The listing builds one solid part. Answer for the finished solid, in the listing's coordinates (mm). A direction names the side the tool comes from. Give positions to 0.01 mm unless a question says otherwise; leave off trailing zeros. Order: outer loops, then holes, each group sorted by start corner. A loop starts at its lowest first (then second) coordinate and runs counter-clockwise, first axis right, second up. Notation, with made-up numbers: (-39.5, 17) - (0.5, 17) arc R31 ccw to (0.5, 56) - close; hole circle Ø11 at (33.25, 18). An arc over 180 degrees is marked (long way). Answer in a Markdown table with one row per item.
from build123d import *

# Parameters (mm, degrees)
F0_W     = 80
F0_H     = 67
F0_R     = 2.5
F0_R_2   = 5
F0_R_3   = 4
F0_R_4   = 3.25
F1_DEPTH = 11.5
F2_SIZE2 = 3
F2_SIZE  = 3
F3_R     = 5
F3_R_2   = 3.25
F4_DEPTH = 5.5


with BuildPart() as f1:
    # F0 (on Top) → F1 (new body)
    with BuildSketch(Plane.XY):
        with Locations((40, 33.5)):
            Rectangle(F0_W, F0_H)
        with Locations((10, 10)):
            Circle(F0_R, mode=Mode.SUBTRACT)
        with Locations((20, 10)):
            Circle(F0_R, mode=Mode.SUBTRACT)
        with Locations((30, 10)):
            Circle(F0_R, mode=Mode.SUBTRACT)
        with Locations((12, 25)):
            Circle(F0_R_2, mode=Mode.SUBTRACT)
        with Locations((26, 25)):
            Circle(F0_R_3, mode=Mode.SUBTRACT)
        with Locations((40, 10)):
            Circle(F0_R, mode=Mode.SUBTRACT)
        with Locations((50, 10)):
            Circle(F0_R, mode=Mode.SUBTRACT)
        with Locations((60, 10)):
            Circle(F0_R, mode=Mode.SUBTRACT)
        with Locations((70, 10)):
            Circle(F0_R, mode=Mode.SUBTRACT)
        with Locations((40, 25)):
            Circle(F0_R_2, mode=Mode.SUBTRACT)
        with BuildLine():
            Line((54, 29), (70, 29))
            ThreePointArc((70, 29), (74, 25), (70, 21))
            Line((70, 21), (54, 21))
            ThreePointArc((54, 21), (50, 25), (54, 29))
        make_face(mode=Mode.SUBTRACT)
        with Locations((10, 42)):
            Circle(F0_R_3, mode=Mode.SUBTRACT)
        with Locations((21, 42)):
            Circle(F0_R_3, mode=Mode.SUBTRACT)
        with Locations((35, 42)):
            Circle(F0_R_4, mode=Mode.SUBTRACT)
        with Locations((10, 57)):
            Circle(F0_R, mode=Mode.SUBTRACT)
        with Locations((20, 57)):
            Circle(F0_R, mode=Mode.SUBTRACT)
        with Locations((30, 57)):
            Circle(F0_R, mode=Mode.SUBTRACT)
        with Locations((52, 42)):
            Circle(F0_R_3, mode=Mode.SUBTRACT)
        with Locations((69, 42)):
            Circle(F0_R_2, mode=Mode.SUBTRACT)
        with Locations((40, 57)):
            Circle(F0_R, mode=Mode.SUBTRACT)
        with Locations((50, 57)):
            Circle(F0_R, mode=Mode.SUBTRACT)
        with Locations((60, 57)):
            Circle(F0_R, mode=Mode.SUBTRACT)
        with Locations((70, 57)):
            Circle(F0_R, mode=Mode.SUBTRACT)
    extrude(amount=F1_DEPTH)

    # F2
    f2_edges = [f1.edges().sort_by_distance(p)[0] for p in [
        (31.75, 42, 11.5),
    ]]
    chamfer(f2_edges, length=F2_SIZE, length2=F2_SIZE2)

    # F3 (on face) → F4 (join)
    with BuildSketch(Plane(origin=(0, 0, 0), x_dir=(1, 0, 0), z_dir=(0, 0, -1))):
        with Locations((40, -25)):
            Circle(F3_R)
        with Locations((40, -25)):
            Circle(F3_R_2, mode=Mode.SUBTRACT)
    extrude(amount=-F4_DEPTH)


solid = f1.part
Item 1: Find section D-D on y = 42. Write down the section's boundary in (x, z).
Answer block:
| item | result |
|---|---|
| outline | (0, 0) - (6, 0) - (6, 11.5) - (0, 11.5) - close; (14, 0) - (17, 0) - (17, 11.5) - (14, 11.5) - close; (25, 0) - (31.75, 0) - (31.75, 8.5) - (28.75, 11.5) - (25, 11.5) - close; (38.25, 0) - (48, 0) - (48, 11.5) - (41.25, 11.5) - (38.25, 8.5) - close; (56, 0) - (64, 0) - (64, 11.5) - (56, 11.5) - close; (74, 0) - (80, 0) - (80, 11.5) - (74, 11.5) - close |
Item 2: This flat-tipped pin is pushed along its axis until it touches: P1, Ø10, axis at x = 13, y = 40, coming from the -Z side. Where does it stop, or does it pass through?
Answer block:
| item | result |
|---|---|
| P1 | z = 0 |
Item 3: Consider line 1 (Y direction, x = 40, z = 3.25); line 2 (Y direction, x = 66, z = 4); line 3 (Y direction, x = 26, z = 5.25). Determine where each line is inside the solid, lowest interval first.
Answer block:
| item | result |
|---|---|
| line 1 | 0 to 7.5, 12.5 to 21.75, 28.25 to 54.5, 59.5 to 67 |
| line 2 | 0 to 21, 29 to 38, 46 to 67 |
| line 3 | 0 to 21, 29 to 67 |
Item 4: Find section B-B on x = 15.5. Write down the section's boundary in (y, z).
Answer block:
| item | result |
|---|---|
| outline | (0, 0) - (21.43, 0) - (21.43, 11.5) - (0, 11.5) - close; (28.57, 0) - (67, 0) - (67, 11.5) - (28.57, 11.5) - close |
Item 5: Which of the six approach directions +Z, -Z, +X, -X, +Y, -Y give full straight-line access (tool end or side, diameter ignored) to faces 4 (the face through (50, 25, 6)), 5 (the face through (39, 34, 11.5))?
Answer block:
| item | result |
|---|---|
| face 4 | +Z, -Z |
| face 5 | +Z, +X, -X, +Y, -Y |
Item 6: Determine the mould class of faces 1 (the face through (39, 67, 6)), 2 (the face through (17.5, 57.1, 5.7)), 3 (the face through (80, 33, 6)) for opening direction X: pulls with the +X half, pulls with the -X half, needs draft (parallel to the pull), parting line crosses it, or undercut.
Answer block:
| item | result |
|---|---|
| face 1 | needs draft |
| face 2 | undercut |
| face 3 | pulls with the +X half |
Item 7: Find section C-C on z = 2.5. Count the separate pieces of the cut face and the enclosed holes in it, then the cut area to 3 significant figures.
Answer block:
| item | result |
|---|---|
| separate pieces | 1 |
| enclosed holes | 23 |
| area | 4,480 mm² |
Item 8: Find section A-A on y = 25. Write down the section's boundary in (x, z).
Answer block:
| item | result |
|---|---|
| outline | (0, 0) - (7, 0) - (7, 11.5) - (0, 11.5) - close; (17, 0) - (22, 0) - (22, 11.5) - (17, 11.5) - close; (30, 0) - (36.75, 0) - (36.75, 5.5) - (35, 5.5) - (35, 11.5) - (30, 11.5) - close; (43.25, 0) - (50, 0) - (50, 11.5) - (45, 11.5) - (45, 5.5) - (43.25, 5.5) - close; (74, 0) - (80, 0) - (80, 11.5) - (74, 11.5) - close |
